Part print with two shaded views. Sizes in mm from the minimum x, y, z corner. A direction names the side the tool comes from. Give positions to 0.01 mm unless a question says otherwise; leave off trailing zeros. Write each loop counter-clockwise with the first axis right and the second up, starting at its lowest first coordinate (ties: lowest second). Pieces come first, ordered by that corner, then holes.
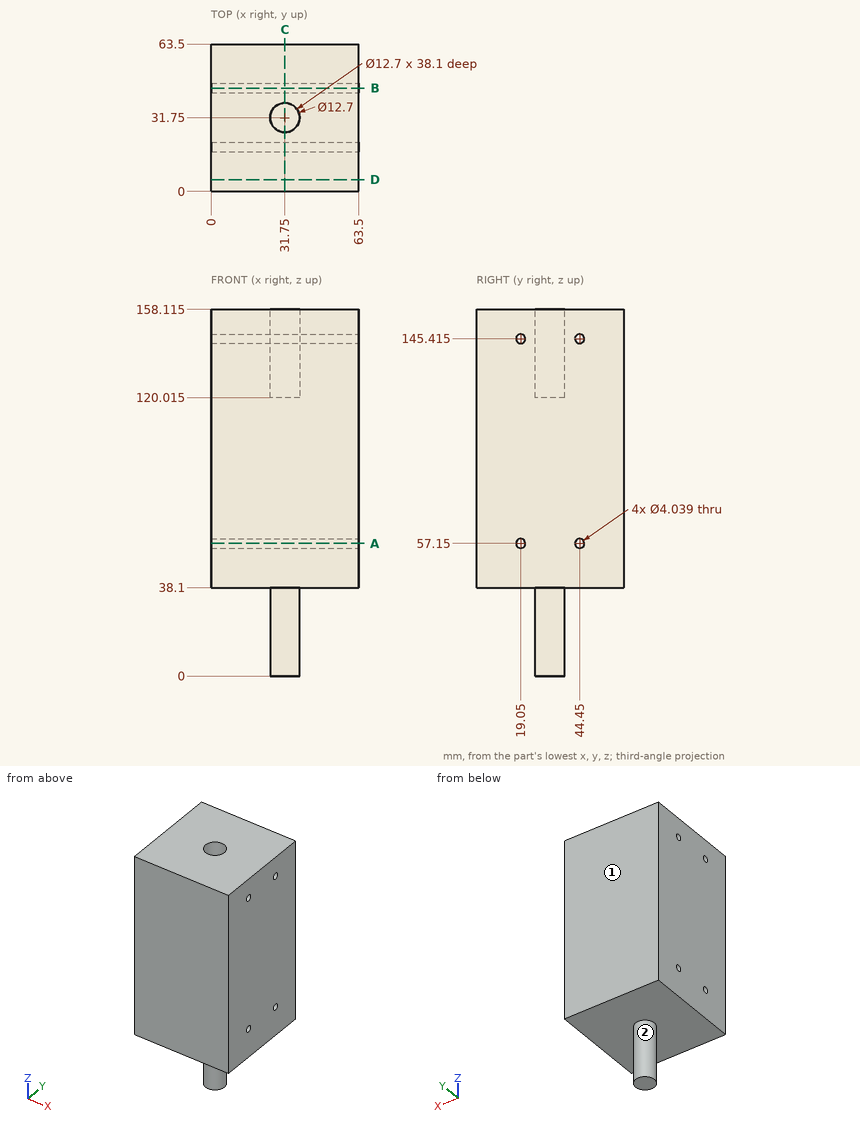
1) Wall check: L1, parallel to Z at x = 19, y = 19 (1 decimal); L2, parallel to Y at x = 29, z = 57; L3, parallel to Z at x = 17.5, y = 17.5 (1 decimal). Give the ranges that are in metal, low to high.
Answers follow:
L1: z = 38.1 to 55.1, 59.2 to 143.4, 147.4 to 158.1
L2: y = 0 to 17.04, 21.06 to 42.44, 46.46 to 63.5
L3: z = 38.1 to 55.9, 58.4 to 144.1, 146.7 to 158.1
2) Saw through at C-C, the plane x = 31.75. Count the separate pieces of the cut face and the enclosed holes in it, then the cut area to 3 significant figures.
Answers follow:
separate pieces: 1
enclosed holes: 4
area: 7,570 mm2
3) Pin check, flat tips, straight feed: pin 1 Ø8 at (x, y) = (19, 41) entering from -Z; pin 2 Ø11.5 at (x, y) = (31.75, 31.75) entering from +Z (3 decimals); pin 3 Ø3.5 at (y, z) = (44.45, 57.15) entering from +X. Stop position of each tip, or through.
Answers follow:
pin 1: stops at z = 38.1
pin 2: stops at z = 120.015
pin 3: passes through
4) Saw through at D-D, the plane y = 5. Write the cut outline in (x, z) (1 decimal).
Answers follow:
outline: (0, 38.1) - (63.5, 38.1) - (63.5, 158.1) - (0, 158.1) - close
5) 3-axis set-ups, long thin cutter, end or side, ignore diameter. For the marked faces 1 and 2: which of +Z, -Z, +X, -X, +Y, -Y reach the whole face in a straight line?
Answers follow:
face 1: +Z, -Z, +X, -X, +Y
face 2: -Z
6) Saw through at B-B, the plane y = 44.45. Write the cut outline in (x, z) (1 decimal), then the cut area to 3 significant figures.
Answers follow:
outline: (0, 38.1) - (63.5, 38.1) - (63.5, 55.1) - (0, 55.1) - close; (0, 59.2) - (63.5, 59.2) - (63.5, 143.4) - (0, 143.4) - close; (0, 147.4) - (63.5, 147.4) - (63.5, 158.1) - (0, 158.1) - close
area: 7,110 mm2
7) Saw through at A-A, the plane z = 57.15. Write the cut outline in (x, y), then the cut area to 3 significant figures.
Answers follow:
outline: (0, 0) - (63.5, 0) - (63.5, 17.03) - (0, 17.03) - close; (0, 21.07) - (63.5, 21.07) - (63.5, 42.43) - (0, 42.43) - close; (0, 46.47) - (63.5, 46.47) - (63.5, 63.5) - (0, 63.5) - close
area: 3,520 mm2
